Part model, mm, in its own coordinate system. Face numbers are marked on the shaded views. A direction names the side the tool comes from. Round coordinates to 2 decimals unless told otherwise and drop trailing zeros. Write each loop counter-clockwise with the first axis right and the second up, starting at its lowest first coordinate (ties: lowest second). Pieces come first, ordered by that corner, then holes. Notation, with made-up numbers: (0, -29.5) -> (54, -29.5) arc R9 cw to (54, -23.5) -> close; hole circle Ø4 at (-29, -37.5). An arc over 180 degrees is marked (long way). Return JSON: item names as keys, results as strings. Group by question number.
(1) Drop flat-ended pins along their axis: pin 1 Ø1.8 at (y, z) = (25.5, -4.5) entering from +X; pin 2 Ø7 at (x, y) = (2.25, 7) entering from -Z; pin 3 Ø1.5 at (x, z) = (-1, -8) entering from -Y; pin 4 Ø5 at (y, z) = (9.5, 5.5) entering from +X. Give the stop position or say it passes through.
(2) Saw through at D-D (x = -2.25). List the corners of the cut face in (y, z).
(3) Saw through at B-B (x = 2.25). List the corners of the cut face in (y, z).
(4) Saw through at A-A (y = 7). List the corners of the cut face in (x, z).
(5) Mould opens along Y. For the marked faces 3, 4 and 5 say: +Y half, -Y half, draft (parallel to the pull), parting line (faces both ways), or undercut.
(6) Tool access for the marked faces 1 and 2: list every direction of +Z, -Z, +X, -X, +Y, -Y with a clear straight run to the whole face (end or side of a thin tool).
(7) Drill centre lines: L1, parallel to Z at x = 5.5, y = 2; L2, parallel to Y at x = -1, z = 9.75; L3, parallel to X at y = 7, z = 14. Where is each one in solid material? Low to high. Write a range as from..to.
(8) Saw through at C-C (z = 8.5). List the corners of the cut face in (x, y).
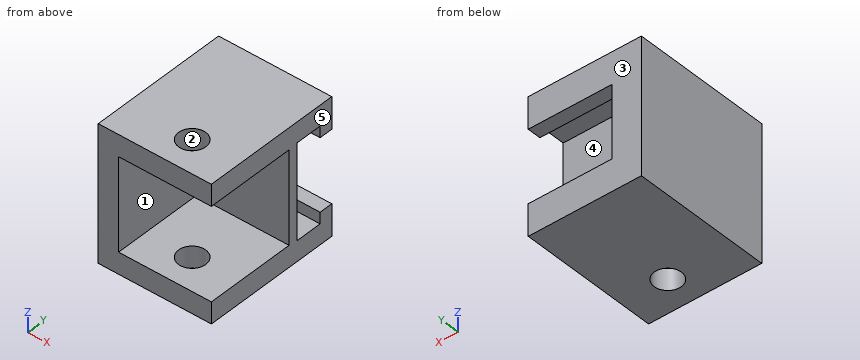
Autodesk Inventor part; units mm, degrees
ref_plane "YZ Plane" through (0, 0, 0) normal (1, 0, 0) x (0, 1, 0)
ref_plane "XZ Plane" through (0, 0, 0) normal (0, 1, 0) x (-1, 0, 0)
ref_plane "XY Plane" through (0, 0, 0) normal (0, 0, 1) x (1, 0, 0)
sketch "スケッチ1" plane through (0, 0, 0) normal (0, 1, 0) x (-1, 0, 0)
  line L0 (-12.5, -15) -> (12.5, -15)
  line L1 (12.5, -15) -> (12.5, 15)
  line L2 (12.5, 15) -> (-12.5, 15)
  line L3 (-12.5, 15) -> (-12.5, -15)
  line L4 (-12.5, -15) -> (12.5, 15) construction
  line L5 (12.5, -15) -> (-12.5, 15) construction
  point P0 (0, 0)
  dimension "d0" = 25
  dimension "d1" = 30
extrude "押し出し1" add sketch "スケッチ1" along normal blind 25
sketch "スケッチ2" plane through (0, 0, 0) normal (0, -1, 0) x (1, 0, 0)
  line L0 (12.5, 15) -> (12.5, -15)
  line L1 (12.5, -10.25) -> (-8, -10.25)
  line L2 (-8, -10.25) -> (-8, 10.25)
  line L3 (-8, 10.25) -> (12.5, 10.25)
  line L4 (12.5, 10.25) -> (12.5, -10.25)
  line L5 (12.5, -15) -> (-12.5, -15)
  point P0 (0, 0)
  point P1 (12.5, 10.25)
  dimension "d4" = 20.5
  dimension "d5" = 20.5
  dimension "d22" = 10.25
extrude "押し出し2" cut sketch "スケッチ2" against normal blind 20
sketch "スケッチ4" plane through (12.5, 0, -15) normal (0, 0, -1) x (-1, 0, 0)
  line L0 (0, 0) -> (25, 0)
  line L1 (0, 0) -> (0, 25)
  point P0 (12.5, 0)
  point P1 (10.25, 7)
  dimension "d12" = 7
  dimension "d13" = 10.25
hole "穴1" at (2.25, 7, -15) direction (0, 0, 1) diameter 6 end through all
sketch "スケッチ6" plane through (0, 25, 0) normal (0, 1, 0) x (1, 0, 0)
  line L0 (-12.5, 15) -> (-12.5, -15)
  line L1 (12.5, -15) -> (12.5, -10.25)
  line L2 (-12.5, 15) -> (12.5, 15)
  line L3 (12.5, 15) -> (12.5, -15)
  line L4 (12.5, -15) -> (-12.5, -15)
  line L5 (-12.5, -15) -> (-12.5, 15)
  point P0 (0, 0)
extrude "押し出し5" add sketch "スケッチ6" along normal blind 6
sketch "スケッチ8" plane through (12.5, 0, -10.25) normal (1, 0, 0) x (0, 0, -1)
  line L0 (-20.75, 28) -> (0.25, 28)
  line L1 (0.25, 28) -> (0.25, 22)
  line L2 (0.25, 22) -> (-20.75, 22)
  line L3 (-20.75, 22) -> (-20.75, 28)
  line L4 (-20.5, 20) -> (0, 20)
  point P0 (-10.25, 0)
  dimension "d37" = 21
  dimension "d38" = 6
  dimension "d39" = 10.5
  dimension "d40" = 2
extrude "押し出し7" cut sketch "スケッチ8" against normal blind 21
sketch "スケッチ9" plane through (12.5, 0, -10.25) normal (1, 0, 0) x (0, 0, -1)
  line L0 (-18.25, 31) -> (-2.25, 31)
  line L1 (-2.25, 31) -> (-2.25, 28)
  line L2 (-2.25, 28) -> (-18.25, 28)
  line L3 (-18.25, 28) -> (-18.25, 31)
  line L4 (-25.25, 31) -> (4.75, 31)
  point P0 (-10.25, 0)
  dimension "d43" = 16
  dimension "d44" = 3
  dimension "d45" = 0
  dimension "d46" = 8
extrude "押し出し8" cut sketch "スケッチ9" against normal blind 18.5
properties part number "baseA"
Computed values:
{
 "1": {"pin 1": "x = -8.5", "pin 2": "z = -15", "pin 3": "y = 20", "pin 4": "x = -8"},
 "2": {"outline": "(0, -15) -> (31, -15) -> (31, -8) -> (28, -8) -> (28, -10.5) -> (22, -10.5) -> (22, 10.5) -> (28, 10.5) -> (28, 8) -> (31, 8) -> (31, 15) -> (0, 15) -> (0, 10.25) -> (20, 10.25) -> (20, -10.25) -> (0, -10.25) -> close"},
 "3": {"outline": "(0, -15) -> (4, -15) -> (4, -10.25) -> (0, -10.25) -> close; (0, 10.25) -> (4, 10.25) -> (4, 15) -> (0, 15) -> close; (10, -15) -> (31, -15) -> (31, -8) -> (28, -8) -> (28, -10.5) -> (22, -10.5) -> (22, 10.5) -> (28, 10.5) -> (28, 8) -> (31, 8) -> (31, 15) -> (10, 15) -> (10, 10.25) -> (20, 10.25) -> (20, -10.25) -> (10, -10.25) -> close"},
 "4": {"outline": "(-12.5, -15) -> (-0.75, -15) -> (-0.75, -10.25) -> (-8, -10.25) -> (-8, 10.25) -> (-0.75, 10.25) -> (-0.75, 15) -> (-12.5, 15) -> close; (5.25, -15) -> (12.5, -15) -> (12.5, -10.25) -> (5.25, -10.25) -> close; (5.25, 10.25) -> (12.5, 10.25) -> (12.5, 15) -> (5.25, 15) -> close"},
 "5": {"face 3": "+Y half", "face 4": "undercut", "face 5": "draft"},
 "6": {"face 1": "+X, -Y", "face 2": "+Z, -Z"},
 "7": {"L1": "-15..-10.25, 10.25..15", "L2": "20..22, 28..31", "L3": "-12.5..-0.75, 5.25..12.5"},
 "8": {"outline": "(-12.5, 0) -> (-8, 0) -> (-8, 20) -> (12.5, 20) -> (12.5, 22) -> (-8.5, 22) -> (-8.5, 28) -> (12.5, 28) -> (12.5, 31) -> (-12.5, 31) -> close"}
}
